from build123d import *

# Parameters (mm, degrees)
SKETCH1_W                      = 190
SKETCH1_H                      = 170
BASE_FLANGE1_DEPTH             = 1
SKETCH23_R                     = 2.5
CUT_EXTRUDE1_DEPTH             = 10
EDGE_FLANGE5_STRIP_W           = 6
EDGE_FLANGE5_STRIP_H           = 1
EDGE_FLANGE5_STRIP_CUT_DEPTH   = 190
EDGE_FLANGE5_STRIP_2_W         = 6
EDGE_FLANGE5_STRIP_2_H         = 1
EDGE_FLANGE5_STRIP_CUT_2_DEPTH = 190
EDGE_FLANGE5_DEPTH             = 190
EDGE_FLANGE5_BEND_DEPTH        = 190
SKETCH44_R                     = 2.5
CUT_EXTRUDE2_DEPTH             = 180


# Sheet-metal steps are written as plain solids
with BuildPart() as part:
    # Sketch1 → Base-Flange1 (new body)
    with BuildSketch(Plane.XY):
        Rectangle(SKETCH1_W, SKETCH1_H)
    extrude(amount=-BASE_FLANGE1_DEPTH)

    # Sketch23 → Cut-Extrude1 (cut)
    with BuildSketch(Plane.XY):
        with Locations((-88, 60)):
            Circle(SKETCH23_R)
        with Locations((88, 60)):
            Circle(SKETCH23_R)
        with Locations((88, -60)):
            Circle(SKETCH23_R)
        with Locations((-88, -60)):
            Circle(SKETCH23_R)
    extrude(amount=-CUT_EXTRUDE1_DEPTH, mode=Mode.SUBTRACT)

    # Edge-Flange5 strip (across the edge) → Edge-Flange5 strip cut (cut)
    with BuildSketch(Plane(origin=(-95, 85, -1), x_dir=(0, -1, 0), z_dir=(1, 0, 0))):
        with Locations((-1, -0.5)):
            Rectangle(EDGE_FLANGE5_STRIP_W, EDGE_FLANGE5_STRIP_H)
    extrude(amount=EDGE_FLANGE5_STRIP_CUT_DEPTH, mode=Mode.SUBTRACT)

    # Edge-Flange5 strip 2 (across the edge) → Edge-Flange5 strip cut 2 (cut)
    with BuildSketch(Plane(origin=(95, -85, -1), x_dir=(0, 1, 0), z_dir=(-1, 0, 0))):
        with Locations((-1, -0.5)):
            Rectangle(EDGE_FLANGE5_STRIP_2_W, EDGE_FLANGE5_STRIP_2_H)
    extrude(amount=EDGE_FLANGE5_STRIP_CUT_2_DEPTH, mode=Mode.SUBTRACT)

    # Edge-Flange5 section (across the edge) → Edge-Flange5 (add)
    with BuildSketch(Plane(origin=(-95, 85, -1), x_dir=(0, -1, 0), z_dir=(1, 0, 0))):
        with BuildLine():
            Line((0, 1), (0, 199))
            Line((0, 199), (1, 199))
            Line((1, 199), (1, 1))
            ThreePointArc((1, 1), (1.292893219, 0.292893219), (2, 0))
            Line((2, 0), (2, -1))
            ThreePointArc((2, -1), (0.585786438, -0.414213562), (0, 1))
        make_face()
    extrude(amount=EDGE_FLANGE5_DEPTH)

    # Edge-Flange5 section 2 (across the edge) → Edge-Flange5 bend (add)
    with BuildSketch(Plane(origin=(95, -85, -1), x_dir=(0, 1, 0), z_dir=(-1, 0, 0))):
        with BuildLine():
            Line((0, 1), (0, 199))
            Line((0, 199), (1, 199))
            Line((1, 199), (1, 1))
            ThreePointArc((1, 1), (1.292893219, 0.292893219), (2, 0))
            Line((2, 0), (2, -1))
            ThreePointArc((2, -1), (0.585786438, -0.414213562), (0, 1))
        make_face()
    extrude(amount=EDGE_FLANGE5_BEND_DEPTH)

    # Sketch44 → Cut-Extrude2 (cut)
    with BuildSketch(Plane(origin=(0, 85, 0), x_dir=(1, 0, 0), z_dir=(0, 1, 0))):
        with Locations(Location((-88, 175, 0), (0, 0, 270))):
            Circle(SKETCH44_R)
        with Locations(Location((88, 175, 0), (0, 0, 270))):
            Circle(SKETCH44_R)
        with Locations(Location((88, 25, 0), (0, 0, 270))):
            Circle(SKETCH44_R)
        with Locations(Location((-88, 25, 0), (0, 0, 270))):
            Circle(SKETCH44_R)
    extrude(amount=-CUT_EXTRUDE2_DEPTH, mode=Mode.SUBTRACT)


solid = part.part
Verification items for the finished model (mm, model axes). A direction names the side the tool comes from. Give positions to 0.01 mm unless a question says otherwise; leave off trailing zeros. Write each loop counter-clockwise with the first axis right and the second up, starting at its lowest first coordinate (ties: lowest second). Pieces come first, ordered by that corner, then holes. Notation, with made-up numbers: M 32,89 L 38,89 A30 cw 38,118 Z; hole C 74,69.25 d8. An arc over 180 degrees is marked long. Write item = value, one per line.
(1) Material ranges on line 1 (X direction, y = -84.6, z = -25); line 2 (Y direction, x = -62, z = -30.5); line 3 (Z direction, x = -45.5, y = 71.5), recorded low to high.
Found:
line_1 = -95 to -90.5, -85.5 to 85.5, 90.5 to 95
line_2 = -85 to -84, 84 to 85
line_3 = -1 to 0
(2) Sectioned sample at B-B (x = 25). Record the cut outline in (y, z).
Found:
outline = M -85,-200 L -84,-200 L -84,-2 A1 cw -83,-1 L 83,-1 A1 cw 84,-2 L 84,-200 L 85,-200 L 85,-2 A2 ccw 83,0 L -83,0 A2 ccw -85,-2 Z
(3) Draft check along X on faces 1 (the face through (-85.52, -84.49, -25.33)), 2 (the face through (1, -85, -100)). Enter one of: released by +X, released by -X, zero draft, split by the parting line, or undercut.
Found:
face_1 = undercut
face_2 = zero draft
(4) Access from +Z, -Z, +X, -X, +Y, -Y to the whole of each face (thin tool, end or side, straight path). Record for faces 3 (the face through (-1, 1, 0)), 4 (the face through (-1, 84, -102)).
Found:
face_3 = +Z, +X, -X, +Y, -Y
face_4 = -Z, +X, -X
(5) Sectioned sample at A-A (z = -17). Record the cut outline in (x, y), then the cut area to 3 significant figures.
Found:
outline = M -95,-85 L 95,-85 L 95,-84 L -95,-84 Z; M -95,84 L 95,84 L 95,85 L -95,85 Z
area = 380 mm2
(6) Go/stop test with a flat-tipped pin: pin 1 Ø8 at (x, y) = (88, 60) entering from -Z. Record where the tip stops, or that it passes through.
Found:
pin_1 = -1
(7) Sectioned sample at C-C (y = 71.5). Record the cut outline in (x, z).
Found:
outline = M -95,-1 L 95,-1 L 95,0 L -95,0 Z
